Read the model definition and answer for the solid it produces. Units are mm, in the model's axes. Coordinates: 2 decimals unless noted, no trailing zeros. Order: outer loops, then holes, each group sorted by start corner. A loop starts at its lowest first (then second) coordinate and runs counter-clockwise, first axis right, second up. Notation, with made-up numbers: (21, 18.5) - (76, 18.5) arc R31 cw to (76, 57.5) - close; hole circle Ø1 at (-1, -21.5). An arc over 180 degrees is marked (long way). Use one line per item in the form item = value.
```python
from build123d import *

# Parameters (mm, degrees)
F1_DEPTH = 1.2


with BuildPart() as f1:
    # F0 (on Top) → F1 (new body)
    with BuildSketch(Plane.XY):
        with BuildLine():
            Line((-30, -50), (30, -50))
            ThreePointArc((30, -50), (33.535534, -48.535534), (35, -45))
            Line((35, -45), (35, 35))
            ThreePointArc((35, 35), (33.535534, 38.535534), (30, 40))
            Line((30, 40), (-5, 40))
            Line((-5, 40), (-5, 45))
            ThreePointArc((-5, 45), (-6.464466, 48.535534), (-10, 50))
            Line((-10, 50), (-30, 50))
            ThreePointArc((-30, 50), (-33.535534, 48.535534), (-35, 45))
            Line((-35, 45), (-35, -45))
            ThreePointArc((-35, -45), (-33.535534, -48.535534), (-30, -50))
        make_face()
    extrude(amount=F1_DEPTH)


solid = f1.part
```
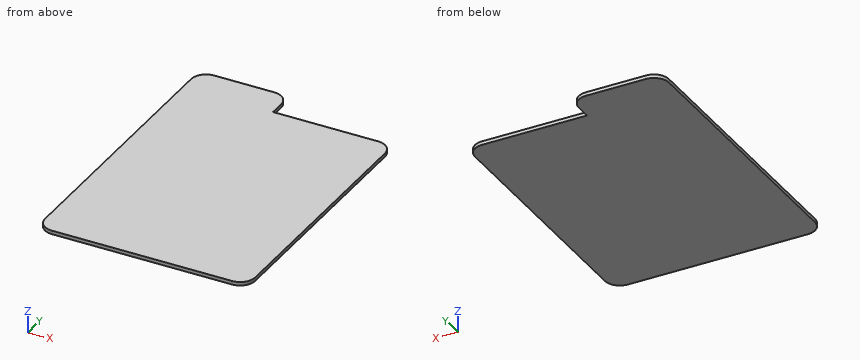
(1) Straight lines are drawn through the part: L1, parallel to Y at x = 19.5, z = 0.2; L2, parallel to X at y = 43, z = 1.15; L3, parallel to Y at x = -6, z = 0.6. For each, find the intervals that lie inside material, in ascending order.
Answer list:
L1 = -50 to 40
L2 = -35 to -5
L3 = -50 to 48
(2) Section B-B, the plane x = 29 is taken. Write down the section's boundary in (y, z).
Answer list:
outline = (-50, 0) - (40, 0) - (40, 1.2) - (-50, 1.2) - close
(3) Section A-A, the plane z = 1 is taken. Write down the section's boundary in (x, y), then the cut area to 3 significant figures.
Answer list:
outline = (-35, -45) arc R5 ccw to (-30, -50) - (30, -50) arc R5 ccw to (35, -45) - (35, 35) arc R5 ccw to (30, 40) - (-5, 40) - (-5, 45) arc R5 ccw to (-10, 50) - (-30, 50) arc R5 ccw to (-35, 45) - close
area = 6,570 mm2
(4) Section C-C, the plane y = 41 is taken. Write down the section's boundary in (x, z).
Answer list:
outline = (-35, 0) - (-5, 0) - (-5, 1.2) - (-35, 1.2) - close
